Geometry check sheet. Reference: the model listing, model coordinates, mm. A direction names the side the tool comes from. Round coordinates to 2 decimals unless told otherwise and drop trailing zeros. Write each loop counter-clockwise with the first axis right and the second up, starting at its lowest first coordinate (ties: lowest second). Pieces come first, ordered by that corner, then holes. Notation, with made-up numbers: M -17.75,15.5 L 26.25,15.5 A15 cw 26.25,19.5 Z; hole C 87,29 d10. An arc over 180 degrees is marked long. One line per item, written item: value. Start each with the question number.
1. Section check B-B (z = 23). Record the boundary of the cut face in (x, y), and give its area (3 significant figures).
2. Access from +Z, -Z, +X, -X, +Y, -Y to the whole of each face (thin tool, end or side, straight path). Record for faces 1 (the flat face through (-35, 17, 0)), 2 (the cylindrical face through (28, 10, -29)), 3 (the cylindrical face through (29.93, 14.1, 16.64)), 4 (the cylindrical face through (-31, 13, 19)), 5 (the flat face through (-30, 5, 17.5)).
3. Section check A-A (x = 0). Record the boundary of the cut face in (y, z).
4. Release check for a two-part mould opening along Y. For faces 6 (the cylindrical face through (-32.908, 10.601, 25.184)), 7 (the flat face through (-30, 6, -7.5)), 8 (the flat face through (0, 0, -6)) record: pulls with the +Y half, pulls with the -Y half, needs draft (parallel to the pull), parting line crosses it, or undercut.
5. Section check D-D (z = -16.5). Record the boundary of the cut face in (x, y), and give its area (3 significant figures).
6. Depth check by flat-ended pin: P1, Ø3, axis at y = 12.5, z = 1.5, coming from the -X side; P2, Ø2, axis at x = 8, y = 4.5, coming from the -Z side; P3, Ø5, axis at x = -28.5, y = 4, coming from the -Z side; P4, Ø3.5, axis at x = 31, y = 10, coming from the -Z side. Enter the tip coordinate at first touch or a pass-through.
7. Section check C-C (y = 10). Count the separate pieces of the cut face and the enclosed holes in it, and give its area (3 significant figures).
8. Scan lines: probe 1 along X at (y, z) = (10, 18); probe 2 along Y at (x, z) = (-31, 26.25); probe 3 along X at (y, z) = (10, -31.5). Record each from-to range of solid material in increasing order. Write a range as [from, to].
from build123d import *

# Parameters (mm, degrees)
SKETCH_1_R               = 15
EXTRUDE_1_DEPTH          = 20
SKETCH_2_W               = 80.970939558
SKETCH_2_H               = 2
CUT_EXTRUDE_1_DEPTH      = 73.284161474
SKETCH_3_W               = 25
SKETCH_3_H               = 30
CUT_EXTRUDE_2_DEPTH      = 10
FILLET_1_R               = 3
CUT_EXTRUDE_3_DEPTH      = 53
CUT_EXTRUDE_3_DEPTH_BACK = 5
SKETCH_4_R               = 3
SKETCH_5_R               = 2
CUT_EXTRUDE_4_DEPTH      = 69.190908514
SKETCH_6_R               = 3
CUT_EXTRUDE_5_DEPTH      = 3
MIRROR_START             = -35
MIRROR_1_DEPTH           = 10
MIRROR_START_2           = 17.3284275
MIRROR_1_2_OUTLINE_R     = 3
MIRROR_1_2_DEPTH         = 3.1715725
SKETCH_7_R               = 2
CUT_EXTRUDE_6_DEPTH      = 42


with BuildPart() as part:
    # 草图1 → 凸台-拉伸1 (new body)
    with BuildSketch(Plane(origin=(0, 0, 0), x_dir=(1, 0, 0), z_dir=(0, 1, 0))):
        with BuildLine():
            Line((-30, 30), (-35, 30))
            Line((-35, 30), (-35, -30))
            Line((-35, -30), (35, -30))
            Line((35, -30), (35, 30))
            Line((35, 30), (30, 30))
            ThreePointArc((30, 30), (0, 60), (-30, 30))
        make_face()
        with Locations(Location((0, 30, 0), (0, 0, 270))):
            Circle(SKETCH_1_R, mode=Mode.SUBTRACT)
    extrude(amount=EXTRUDE_1_DEPTH)

    # 草图2 → 切除-拉伸1 (cut, through all)
    with BuildSketch(Plane(origin=(0, 20, 0), x_dir=(1, 0, 0), z_dir=(0, 1, 0))):
        with Locations((35, 23.224842932)):
            Rectangle(SKETCH_2_W, SKETCH_2_H)
    extrude(amount=-CUT_EXTRUDE_1_DEPTH, mode=Mode.SUBTRACT)

    # 草图3 → 切除-拉伸2 (cut)
    with BuildSketch(Plane(origin=(35, 0, 0), x_dir=(0, 0, -1), z_dir=(1, 0, 0))):
        with Locations((-5, 0)):
            Rectangle(SKETCH_3_W, SKETCH_3_H)
    extrude(amount=-CUT_EXTRUDE_2_DEPTH, mode=Mode.SUBTRACT)

    # 圆角1
    fillet_1_edges = [part.edges().sort_by_distance(p)[0] for p in [
        (30, 15, -7.5),
        (30, 15, 17.5),
    ]]
    fillet(fillet_1_edges, radius=FILLET_1_R)

    # 草图4 → 切除-拉伸3 (cut, two sides: drawn at the far end of the back side and taken through both)
    with BuildSketch(Plane(origin=(0, 0, -30), x_dir=(-1, 0, 0), z_dir=(0, 0, -1)).offset(-CUT_EXTRUDE_3_DEPTH_BACK)):
        with Locations(Location((-31, 10, 0), (0, 0, 70.528779366))):
            Circle(SKETCH_4_R)
    extrude(amount=CUT_EXTRUDE_3_DEPTH + CUT_EXTRUDE_3_DEPTH_BACK, mode=Mode.SUBTRACT)

    # 草图5 → 切除-拉伸4 (cut, through all)
    with BuildSketch(Plane(origin=(0, 0, -25), x_dir=(-1, 0, 0), z_dir=(0, 0, -1))):
        with Locations((-31, 10)):
            Circle(SKETCH_5_R)
    extrude(amount=-CUT_EXTRUDE_4_DEPTH, mode=Mode.SUBTRACT)

    # 草图6 → 切除-拉伸5 (cut, symmetric)
    with BuildSketch(Plane(origin=(0, 0, 17.5), x_dir=(-1, 0, 0), z_dir=(0, 0, -1))):
        with Locations(Location((-31, 10, 0), (0, 0, 70.528779366))):
            Circle(SKETCH_6_R)
    extrude(amount=CUT_EXTRUDE_5_DEPTH, both=True, mode=Mode.SUBTRACT)

    # 镜向1: read off the stored shape, not the designer's step
    # 镜向1 outline → 镜向1 (cut)
    with BuildSketch(Plane.YZ.offset(MIRROR_START)):
        with BuildLine():
            Line((12, 17.5), (0, 17.5))
            Line((0, 17.5), (0, -7.5))
            Line((0, -7.5), (12, -7.5))
            ThreePointArc((12, -7.5), (14.121320344, -6.621320344), (15, -4.5))
            Line((15, -4.5), (15, 14.5))
            ThreePointArc((15, 14.5), (14.121320344, 16.621320344), (12, 17.5))
        make_face()
    extrude(amount=MIRROR_1_DEPTH, mode=Mode.SUBTRACT)

    # Mirror 1 2 outline → Mirror 1 2 (cut)
    with BuildSketch(Plane.XY.offset(MIRROR_START_2)):
        with Locations((-31, 10)):
            Circle(MIRROR_1_2_OUTLINE_R)
    extrude(amount=MIRROR_1_2_DEPTH, mode=Mode.SUBTRACT)

    # 草图7 → 切除-拉伸6 (cut)
    with BuildSketch(Plane(origin=(0, 0, 20.5), x_dir=(-1, 0, 0), z_dir=(0, 0, -1))):
        with Locations((31, 10)):
            Circle(SKETCH_7_R)
    extrude(amount=-CUT_EXTRUDE_6_DEPTH, mode=Mode.SUBTRACT)


solid = part.part
Result sheet:
1. outline: M -35,0 L 35,0 L 35,20 L -35,20 Z; hole C -31,10 d4; hole C 31,10 d4
1. area: 1,370 mm2
2. face 1: +Z, -Z, -X, +Y, -Y
2. face 2: -Z
2. face 3: +X, -Y
2. face 4: none
2. face 5: -X, -Y
3. outline: M 0,-60 L 20,-60 L 20,-45 L 0,-45 Z; M 0,-15 L 20,-15 L 20,30 L 0,30 Z
4. face 6: undercut
4. face 7: needs draft
4. face 8: pulls with the -Y half
5. outline: M -35,0 L -6.54,0 L -6.54,20 L -35,20 Z; M 6.54,0 L 35,0 L 35,20 L 6.54,20 Z; hole C 31,10 d4
5. area: 1,130 mm2
6. P1: stops at x = -25
6. P2: stops at z = -59.17
6. P3: stops at z = -44.97
6. P4: passes through
7. separate pieces: 5
7. enclosed holes: 0
7. area: 4,150 mm2
8. probe 1: x = [-35, -34], [-28, 28], [34, 35]
8. probe 2: y = [0, 8], [12, 20]
8. probe 3: x = [-29.96, -14.92], [14.92, 28]
